```python
from build123d import *

# Parameters (mm, degrees)
SKETCH1_W           = 77
SKETCH1_H           = 77
BOSS_EXTRUDE1_DEPTH = 5
SKETCH2_W           = 87
SKETCH2_H           = 87
SKETCH2_W_2         = 77
SKETCH2_H_2         = 77
BOSS_EXTRUDE2_DEPTH = 33
SKETCH3_R           = 3.5
SKETCH3_R_2         = 2
BOSS_EXTRUDE4_DEPTH = 18.5
SKETCH11_W          = 1.5
SKETCH11_H          = 28
BOSS_EXTRUDE7_DEPTH = 1.5
BOSS_EXTRUDE8_DEPTH = 4
SKETCH7_R           = 4
CUT_EXTRUDE1_DEPTH  = 2
CUT_EXTRUDE2_DEPTH  = 5
SKETCH16_W          = 10
SKETCH16_H          = 5
CUT_EXTRUDE3_DEPTH  = 5
BOSS_EXTRUDE6_DEPTH = 7.5
FILLET1_R           = 2
FILLET2_R           = 1
CHAMFER1_SIZE       = 3
FILLET3_R           = 2


with BuildPart() as part:
    # Sketch1 → Boss-Extrude1 (new body)
    with BuildSketch(Plane(origin=(0, 0, 0), x_dir=(1, 0, 0), z_dir=(0, 1, 0))):
        Rectangle(SKETCH1_W, SKETCH1_H)
    extrude(amount=BOSS_EXTRUDE1_DEPTH)

    # Sketch2 → Boss-Extrude2 (add)
    with BuildSketch(Plane(origin=(0, 0, 0), x_dir=(1, 0, 0), z_dir=(0, 1, 0))):
        Rectangle(SKETCH2_W, SKETCH2_H)
        Rectangle(SKETCH2_W_2, SKETCH2_H_2, mode=Mode.SUBTRACT)
    extrude(amount=BOSS_EXTRUDE2_DEPTH)

    # Sketch3 → Boss-Extrude4 (add)
    # profile 1 of 4: a face of its own
    with BuildSketch(Plane(origin=(0, 5, 0), x_dir=(1, 0, 0), z_dir=(0, 1, 0))):
        with Locations(Location((-28.5, -19, 0), (0, 0, 90))):
            Circle(SKETCH3_R)
        with Locations(Location((-28.5, -19, 0), (0, 0, 270))):
            Circle(SKETCH3_R_2, mode=Mode.SUBTRACT)
    # profile 2 of 4: a face of its own
    with BuildSketch(Plane(origin=(0, 5, 0), x_dir=(1, 0, 0), z_dir=(0, 1, 0))):
        with Locations(Location((-19, 19, 0), (0, 0, 90))):
            Circle(SKETCH3_R)
        with Locations(Location((-19, 19, 0), (0, 0, 270))):
            Circle(SKETCH3_R_2, mode=Mode.SUBTRACT)
    # profile 3 of 4: a face of its own
    with BuildSketch(Plane(origin=(0, 5, 0), x_dir=(1, 0, 0), z_dir=(0, 1, 0))):
        with Locations(Location((28.5, -19, 0), (0, 0, 90))):
            Circle(SKETCH3_R)
        with Locations(Location((28.5, -19, 0), (0, 0, 270))):
            Circle(SKETCH3_R_2, mode=Mode.SUBTRACT)
    # profile 4 of 4: a face of its own
    with BuildSketch(Plane(origin=(0, 5, 0), x_dir=(1, 0, 0), z_dir=(0, 1, 0))):
        with Locations(Location((19, 19, 0), (0, 0, 90))):
            Circle(SKETCH3_R)
        with Locations(Location((19, 19, 0), (0, 0, 270))):
            Circle(SKETCH3_R_2, mode=Mode.SUBTRACT)
    extrude(amount=BOSS_EXTRUDE4_DEPTH)

    # Sketch11 → Boss-Extrude7 (add)
    with BuildSketch(Plane(origin=(0, 5, 0), x_dir=(1, 0, 0), z_dir=(0, 1, 0))):
        with Locations((4.75, 24.5)):
            Rectangle(SKETCH11_W, SKETCH11_H)
        with Locations((-4.75, 24.5)):
            Rectangle(SKETCH11_W, SKETCH11_H)
    extrude(amount=BOSS_EXTRUDE7_DEPTH)

    # Sketch17 → Boss-Extrude8 (add)
    with BuildSketch(Plane(origin=(0, 5, 0), x_dir=(1, 0, 0), z_dir=(0, 1, 0))):
        Polygon((-8.89, 10.5), (-8.89, 5.5), (8.89, 5.5), (8.89, 10.5), (11.89, 10.5), (11.89, 3), (-11.89, 3), (-11.89, 10.5), align=None)
    extrude(amount=BOSS_EXTRUDE8_DEPTH)

    # Sketch7 → Cut-Extrude1 (cut)
    with BuildSketch(Plane.XZ):
        with Locations(Location((-27.5, -27.5, 0), (0, 0, 270))):
            Circle(SKETCH7_R)
        with Locations(Location((-27.5, 27.5, 0), (0, 0, 270))):
            Circle(SKETCH7_R)
        with Locations(Location((27.5, 27.5, 0), (0, 0, 270))):
            Circle(SKETCH7_R)
        with Locations(Location((27.5, -27.5, 0), (0, 0, 270))):
            Circle(SKETCH7_R)
    extrude(amount=-CUT_EXTRUDE1_DEPTH, mode=Mode.SUBTRACT)

    # Sketch10 → Cut-Extrude2 (cut)
    with BuildSketch(Plane(origin=(0, 0, -38.5), x_dir=(-1, 0, 0), z_dir=(0, 0, -1))):
        with BuildLine():
            Line((-5, 13), (5, 13))
            ThreePointArc((5, 13), (7.5, 10.5), (5, 8))
            Line((5, 8), (-5, 8))
            ThreePointArc((-5, 8), (-7.5, 10.5), (-5, 13))
        make_face()
    extrude(amount=CUT_EXTRUDE2_DEPTH, mode=Mode.SUBTRACT)

    # Sketch16 → Cut-Extrude3 (cut)
    with BuildSketch(Plane.ZY.offset(-38.5)):
        with Locations((-23.5, 7.5)):
            Rectangle(SKETCH16_W, SKETCH16_H)
    extrude(amount=-CUT_EXTRUDE3_DEPTH, mode=Mode.SUBTRACT)

    # Sketch15 → Boss-Extrude6 (add)
    with BuildSketch(Plane(origin=(0, 5, 0), x_dir=(1, 0, 0), z_dir=(0, 1, 0))):
        Polygon((-11, -0.5), (-11, -8.5), (-13, -8.5), (-13, 1.5), (-6, 1.5), (-6, -0.5), align=None)
        Polygon((-13, -24.5), (-11, -24.5), (-11, -32.5), (-6, -32.5), (-6, -34.5), (-13, -34.5), align=None)
        Polygon((13, -24.5), (11, -24.5), (11, -32.5), (6, -32.5), (6, -34.5), (13, -34.5), align=None)
        Polygon((6, 1.5), (6, -0.5), (11, -0.5), (11, -8.5), (13, -8.5), (13, 1.5), align=None)
    extrude(amount=BOSS_EXTRUDE6_DEPTH)

    # Fillet1
    fillet1_edges = [part.edges().sort_by_distance(p)[0] for p in [
        (28.5, 5, 22.5),
        (19, 5, -15.5),
        (-28.5, 5, 22.5),
        (-19, 5, -15.5),
    ]]
    fillet(fillet1_edges, radius=FILLET1_R)

    # Fillet2
    fillet2_edges = [part.edges().sort_by_distance(p)[0] for p in [
        (-8.89, 7, -10.5),
        (-11.89, 7, -10.5),
        (-11.89, 7, -3),
        (11.89, 7, -3),
        (11.89, 7, -10.5),
        (8.89, 7, -10.5),
        (-13, 8.75, -1.5),
        (13, 8.75, -1.5),
        (-13, 8.75, 34.5),
        (13, 8.75, 34.5),
    ]]
    fillet(fillet2_edges, radius=FILLET2_R)

    # Chamfer1
    chamfer1_edges = [part.edges().sort_by_distance(p)[0] for p in [
        (-43.5, 16.5, 43.5),
        (43.5, 16.5, 43.5),
        (43.5, 16.5, -43.5),
        (-43.5, 16.5, -43.5),
    ]]
    chamfer(chamfer1_edges, length=CHAMFER1_SIZE)

    # Fillet3
    fillet3_edges = [part.edges().sort_by_distance(p)[0] for p in [
        (-40.5, 16.5, -43.5),
        (40.5, 16.5, -43.5),
        (43.5, 16.5, 40.5),
        (43.5, 16.5, -40.5),
        (40.5, 16.5, 43.5),
        (-40.5, 16.5, 43.5),
        (-43.5, 16.5, -40.5),
        (-43.5, 16.5, 40.5),
    ]]
    fillet(fillet3_edges, radius=FILLET3_R)


solid = part.part
```
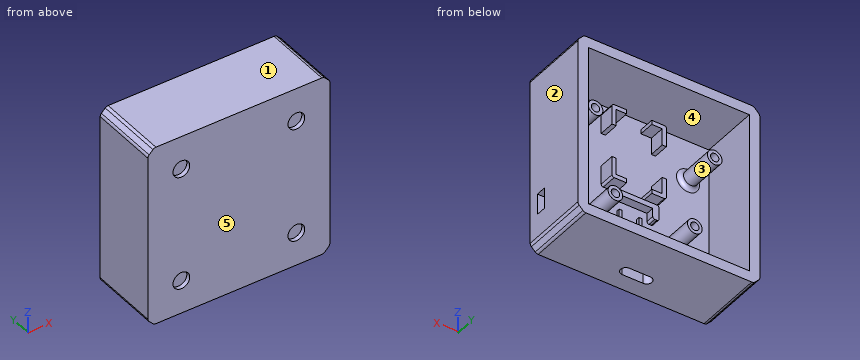
For this review, take the finished solid that the model builds, in its own axes (mm). Face numbers are marked on the shaded views. A direction names the side the tool comes from. Round coordinates to 2 decimals unless told otherwise and drop trailing zeros. Write each loop counter-clockwise with the first axis right and the second up, starting at its lowest first coordinate (ties: lowest second). Pieces come first, ordered by that corner, then holes. Notation, with made-up numbers: M 59.25,7.25 L 67.25,7.25 A22 cw 67.25,26.25 Z; hole C 12.5,-2.75 d2. An arc over 180 degrees is marked long. One line per item, written item: value. Start each with the question number.
(1) We need section D-D (x = -19). Give the boundary of the cut face in (y, z).
(2) We need section C-C (z = 27.5). Give the boundary of the cut face in (x, y).
(3) Insertion check: pin 1 (7.5 mm diameter, centred on x = 10.5, z = 31, fed in from +Y); pin 2 (6.5 mm diameter, centred on x = 28.5, z = -28, fed in from -Y); pin 3 (5 mm diameter, centred on x = 16, z = 30, fed in from +Y); pin 4 (1.5 mm diameter, centred on x = 4.5, y = 10.5, fed in from -Z). Each pin has a flat end and moves straight along its axis. Give the tip position at first contact, or say it passes through.
(4) We need section A-A (x = -37). Give the boundary of the cut face in (y, z).
(5) We need section B-B (y = 25.5). Give the boundary of the cut face in (x, z).
(6) The part is to be moulded in two halves that separate along Z. For the marked faces 1, 2 and 3, say which applies: released by +Z, released by -Z, zero draft, split by the parting line, or undercut.
(7) Wall thickness on line 1 (Z direction, x = -1.5, y = 7); line 2 (Z direction, x = 10.5, y = 9.5); line 3 (X direction, y = 14.5, z = 28): over which ranges is each line inside the solid? List them lowest first.
(8) Machinability: for the marked faces 4 and 5, which of the approach directions +Z, -Z, +X, -X, +Y, -Y give a long, thin tool a straight path to every point of the face, cutting with its end or side? Answer none if there is none.
Result:
1. outline: M 0,-43.5 L 33,-43.5 L 33,-38.5 L 5,-38.5 L 5,-24.5 A2 cw 7,-22.5 L 23.5,-22.5 L 23.5,-21 L 5,-21 L 5,-17 L 23.5,-17 L 23.5,-15.5 L 7,-15.5 A2 cw 5,-13.5 L 5,38.5 L 33,38.5 L 33,43.5 L 0,43.5 Z
2. outline: M -43.5,0 L -31.5,0 L -31.5,2 L -23.5,2 L -23.5,0 L 23.5,0 L 23.5,2 L 31.5,2 L 31.5,0 L 43.5,0 L 43.5,33 L 38.5,33 L 38.5,5 L 13,5 L 13,12.5 L 11,12.5 L 11,5 L -11,5 L -11,12.5 L -13,12.5 L -13,5 L -38.5,5 L -38.5,33 L -43.5,33 Z
3. pin 1: y = 12.5
3. pin 2: y = 0
3. pin 3: y = 5
3. pin 4: z = 38.5
4. outline: M 0,-43.5 L 33,-43.5 L 33,-38.5 L 5,-38.5 L 5,38.5 L 33,38.5 L 33,43.5 L 0,43.5 Z
5. outline: M -43.5,-39.67 A2 ccw -42.91,-41.09 L -41.09,-42.91 A2 ccw -39.67,-43.5 L 39.67,-43.5 A2 ccw 41.09,-42.91 L 42.91,-41.09 A2 ccw 43.5,-39.67 L 43.5,39.67 A2 ccw 42.91,41.09 L 41.09,42.91 A2 ccw 39.67,43.5 L -39.67,43.5 A2 ccw -41.09,42.91 L -42.91,41.09 A2 ccw -43.5,39.67 Z; hole M -38.5,-38.5 L 38.5,-38.5 L 38.5,38.5 L -38.5,38.5 Z
6. face 1: released by +Z
6. face 2: zero draft
6. face 3: undercut
7. line 1: -43.5 to -38.5, -5.5 to -3, 38.5 to 43.5
7. line 2: -43.5 to -38.5, -1.5 to 0.5, 32.5 to 34.5, 38.5 to 43.5
7. line 3: -43.5 to -38.5, 38.5 to 43.5
8. face 4: +Y
8. face 5: +Z, -Z, +X, -X, -Y
